Part model, mm, in its own coordinate system. Face numbers are marked on the shaded views. A direction names the side the tool comes from. Give positions to 0.01 mm unless a question says otherwise; leave off trailing zeros. Order: outer loops, then holes, each group sorted by start corner. A loop starts at its lowest first (then second) coordinate and runs counter-clockwise, first axis right, second up.
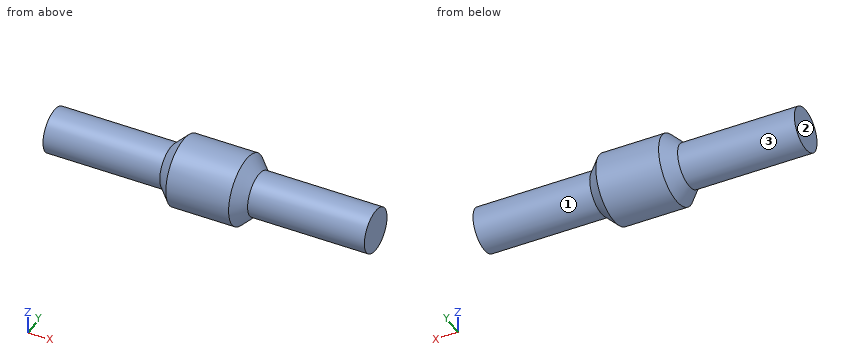
from build123d import *


with BuildPart() as part:
    # Sketch2 → Revolve1 (revolve)
    with BuildSketch(Plane.XY, mode=Mode.PRIVATE) as revolve1_sk:
        Polygon((12.8, 0), (12.8, 1.75), (3.5, 1.75), (2.5, 2.75), (0, 2.75), (0, 0), align=None)
    revolve1 = revolve(revolve1_sk.sketch.rotate(Axis((-20, 0, 0), (1, 0, 0)), 90), axis=Axis((-20, 0, 0), (1, 0, 0)))

    # Mirror1: Revolve1 across plane
    add(revolve1.mirror(Plane(origin=(0, 0, 0), x_dir=(0, 0, 1), z_dir=(1, 0, 0))))


solid = part.part
Item 1: Band-saw the part on A-A on y = 0. List the corners of the cut face in (x, z), plus the area to 3 significant figures.
Item 2: Which spindle directions (+Z, -Z, +X, -X, +Y, -Y) get a long thin tool onto all of the face, cutting with end or side? Do the marked faces 1, 2 and 3. Say none if no direction does.
Item 3: Band-saw the part on C-C on x = 5. List the corners of the cut face in (y, z), plus the area to 3 significant figures.
Item 4: Drill centre lines: probe 1 along Z at (x, y) = (2, 1.15); probe 2 along Y at (x, z) = (6.5, 0.1); probe 3 along Y at (x, z) = (-8.25, -0.65). Where is each one in solid material? Low to high.
Item 5: Drop flat-ended pins along their axis: P1, Ø2, axis at x = 1, y = 2, coming from the -Z side; P2, Ø3, axis at x = 3, y = 2, coming from the +Z side; P3, Ø1.5, axis at x = -1, z = 1.5, coming from the +Y side. Give the stop position or say it passes through.
Working result:
1. outline: (-12.8, -1.75) - (-3.5, -1.75) - (-2.5, -2.75) - (2.5, -2.75) - (3.5, -1.75) - (12.8, -1.75) - (12.8, 1.75) - (3.5, 1.75) - (2.5, 2.75) - (-2.5, 2.75) - (-3.5, 1.75) - (-12.8, 1.75) - close
1. area: 102 mm2
2. face 1: +X
2. face 2: +Z, -Z, -X, +Y, -Y
2. face 3: -X
3. outline: circle Ø3.5 at (0, 0)
3. area: 9.62 mm2
4. probe 1: z = -2.5 to 2.5
4. probe 2: y = -1.75 to 1.75
4. probe 3: y = -1.62 to 1.62
5. P1: stops at z = -2.56
5. P2: stops at z = 2.69
5. P3: stops at y = 2.65
